Geometry: see drawing. Coordinates: mm, zero at the bounding-box minimum. Give positions to 0.01 mm unless a question says otherwise; leave off trailing zeros. Write each loop counter-clockwise with the first axis right and the second up, starting at its lowest first coordinate (ties: lowest second). Pieces come first, ordered by that corner, then holes. Notation, with made-up numbers: (-3.5, -34) - (21.5, -34) arc R20 ccw to (21.5, -2) - close; hole circle Ø7 at (7.25, 89.25). An arc over 180 degrees is marked (long way). One line per question, with ' | ' between items. Start each with the question number.
(1) Section D-D, the plane z = 133. Return loops of the section in (x, y).
(2) Section B-B, the plane x = 44.45. Return loops of the section in (y, z), plus the area to 3 significant figures.
(3) Section A-A, the plane z = 38.1. Return loops of the section in (x, y).
(4) Section C-C, the plane x = 8. Return loops of the section in (y, z), plus the area to 3 significant figures.
(5) Pin query (flat end, axial travel): pin 1 (7 mm diameter, centred on y = 4, z = 116.5, fed in from +X); pin 2 (1.9 mm diameter, centred on y = 4, z = 121, fed in from -X); pin 3 (2 mm diameter, centred on y = 14.5, z = 118, fed in from +X); pin 4 (20.5 mm diameter, centred on x = 44.45, z = 114.3, fed in from -Y). Return the tip coordinate at first contact, or that it passes through.
(6) Draft query along Z for the marked faces 1, 2 and 3. Return one class per face: +Z half, -Z half, draft (parallel to the pull), parting line (faces both ways), or undercut.
(7) Ray query, line 1 (Z direction, x = 44.45, y = 16.25); line 2 (Z direction, x = 46, y = 2.5); line 3 (X direction, y = 4.25, z = 115.5). Return the intervals inside material, ascending. Write a range as [from, to].
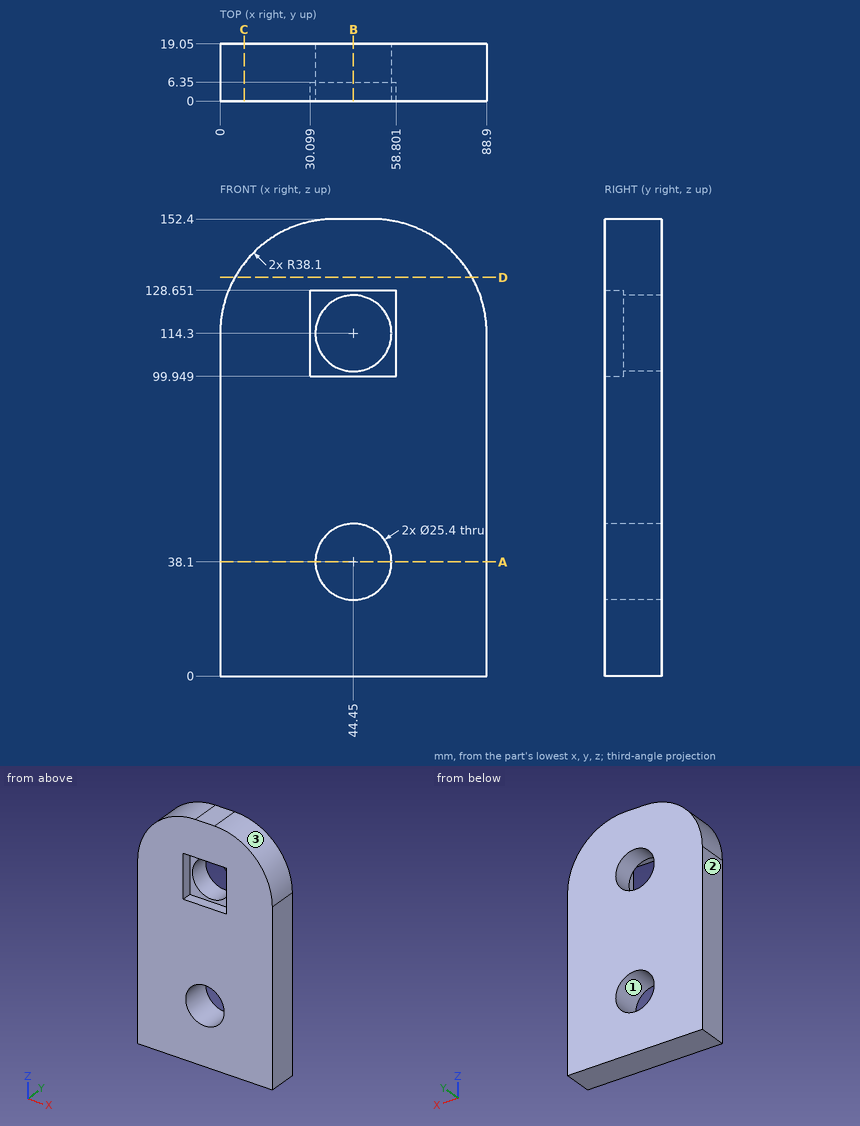
Check sheet entries:
1) outline: (4.9, 0) - (84, 0) - (84, 19.05) - (4.9, 19.05) - close
2) outline: (0, 0) - (19.05, 0) - (19.05, 25.4) - (0, 25.4) - close; (0, 50.8) - (19.05, 50.8) - (19.05, 101.6) - (6.35, 101.6) - (6.35, 99.95) - (0, 99.95) - close; (0, 128.65) - (6.35, 128.65) - (6.35, 127) - (19.05, 127) - (19.05, 152.4) - (0, 152.4) - close | area: 1,910 mm²
3) outline: (0, 0) - (31.75, 0) - (31.75, 19.05) - (0, 19.05) - close; (57.15, 0) - (88.9, 0) - (88.9, 19.05) - (57.15, 19.05) - close
4) outline: (0, 0) - (19.05, 0) - (19.05, 137.66) - (0, 137.66) - close | area: 2,620 mm²
5) pin 1: x = 88.9 | pin 2: x = 0.44 | pin 3: x = 88.8 | pin 4: through
6) face 1: undercut | face 2: draft | face 3: +Z half
7) line 1: [0, 25.4], [50.8, 101.6], [127, 152.4] | line 2: [0, 25.49], [50.71, 99.95], [128.65, 152.4] | line 3: [0.02, 30.1], [58.8, 88.88]
